Check sheet for the drawn part. Datum: minimum x, y, z corner. Units: mm. Round coordinates to 2 decimals unless told otherwise and drop trailing zeros. Write each loop counter-clockwise with the first axis right and the second up, starting at its lowest first coordinate (ties: lowest second). Pieces come first, ordered by that corner, then holes.
Item 1: Cross-section at C-C on z = 54.5. Enter the section's corners in (x, y).
Item 2: Cross-section at A-A on y = 0.7. Enter the section's corners in (x, z).
Item 3: Go/stop test with a flat-tipped pin: pin 1 Ø0.6 at (x, y) = (48, 1) entering from +Z. Record where the tip stops, or that it passes through.
Item 4: Material ranges on line 1 (Z direction, x = 48.5, y = 1.5); line 2 (X direction, y = 1.7, z = 9.5); line 3 (X direction, y = 1.55, z = 3.5), recorded low to high.
Item 5: Cross-section at B-B on x = 49. Enter the section's corners in (y, z).
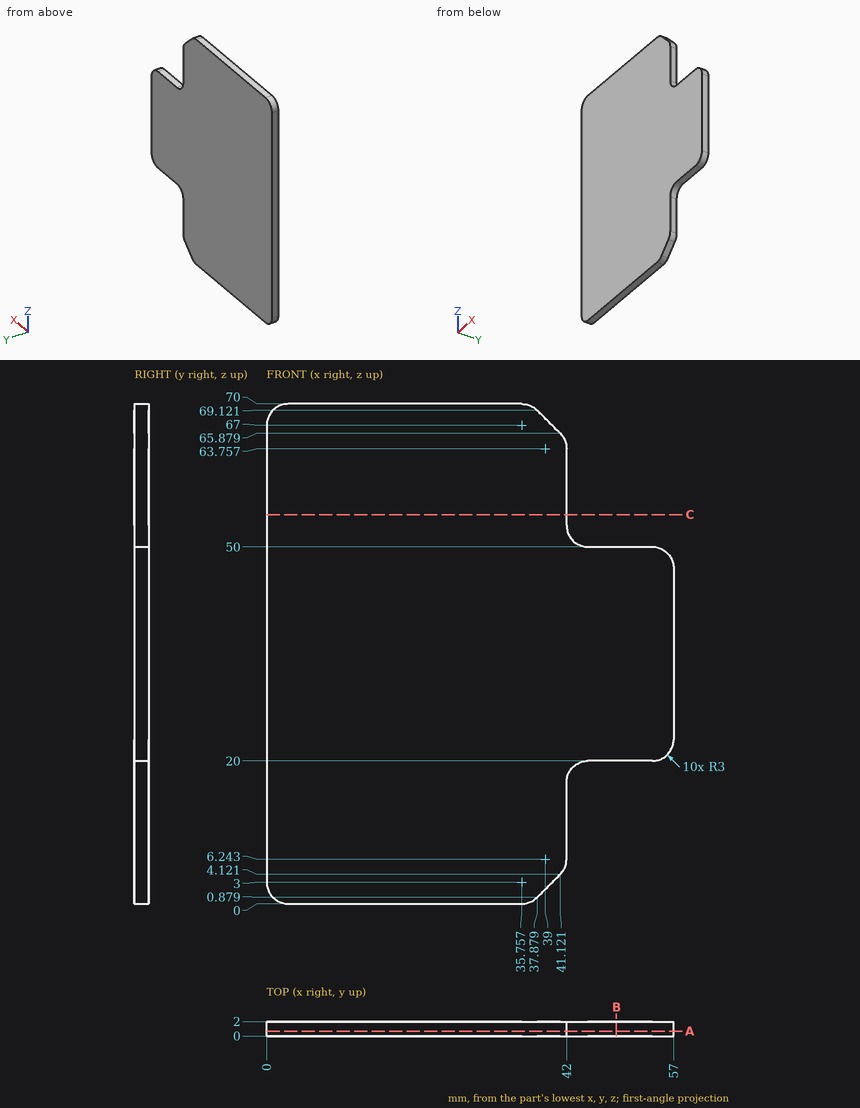
Response values:
1. outline: (0, 0) - (42, 0) - (42, 2) - (0, 2) - close
2. outline: (0, 3) arc R3 ccw to (3, 0) - (35.76, 0) arc R3 ccw to (37.88, 0.88) - (41.12, 4.12) arc R3 ccw to (42, 6.24) - (42, 17) arc R3 cw to (45, 20) - (54, 20) arc R3 ccw to (57, 23) - (57, 47) arc R3 ccw to (54, 50) - (45, 50) arc R3 cw to (42, 53) - (42, 63.76) arc R3 ccw to (41.12, 65.88) - (37.88, 69.12) arc R3 ccw to (35.76, 70) - (3, 70) arc R3 ccw to (0, 67) - close
3. pin 1: stops at z = 50
4. line 1: z = 20 to 50
4. line 2: x = 0 to 42
4. line 3: x = 0 to 40.5
5. outline: (0, 20) - (2, 20) - (2, 50) - (0, 50) - close
